Autodesk Inventor part; units mm, degrees
ref_plane "YZ Plane" through (0, 0, 0) normal (1, 0, 0) x (0, 1, 0)
ref_plane "XZ Plane" through (0, 0, 0) normal (0, 1, 0) x (-1, 0, 0)
ref_plane "XY Plane" through (0, 0, 0) normal (0, 0, 1) x (1, 0, 0)
sketch "스케치1" plane through (0, 0, 0) normal (0, 1, 0) x (-1, 0, 0)
  line L0 (0, 0) -> (106, 0)
  line L1 (106, 0) -> (106, -67)
  line L2 (106, -67) -> (0, -67)
  line L3 (0, -67) -> (0, 0)
  circle A0 centre (5, -15) radius 1.1
  circle A1 centre (5, -31) radius 1.1
  circle A2 centre (5, -47) radius 1.1
  circle A3 centre (101, -15) radius 1.1
  circle A4 centre (101, -31) radius 1.1
  circle A5 centre (101, -47) radius 1.1
  dimension "d1" = 2.2
  dimension "d4" = 16
  dimension "d7" = 96
  dimension "d10" = 5
  dimension "d11" = 15
  dimension "d12" = 5
  dimension "d13" = 20
extrude "돌출1" add sketch "스케치1" along normal blind 5
sketch "스케치2" plane through (0, 5, 0) normal (0, 1, 0) x (1, 0, 0)
  circle A0 centre (-5, 15) radius 1.1
  circle A1 centre (-5, 15) radius 2.1
  circle A2 centre (-5, 31) radius 1.1
  circle A3 centre (-5, 31) radius 2.1
  circle A4 centre (-5, 47) radius 1.1
  circle A5 centre (-5, 47) radius 2.1
  circle A6 centre (-101, 47) radius 1.1
  circle A7 centre (-101, 47) radius 2.1
  circle A8 centre (-101, 31) radius 1.1
  circle A9 centre (-101, 31) radius 2.1
  circle A10 centre (-101, 15) radius 1.1
  circle A11 centre (-101, 15) radius 2.1
  point P0 (0, 0)
  dimension "d16" = 4.2
  dimension "d17" = 4.2
  dimension "d18" = 4.2
  dimension "d19" = 4.2
  dimension "d20" = 4.2
  dimension "d21" = 4.2
extrude "돌출2" cut sketch "스케치2" against normal blind 3
sketch "스케치3" plane through (0, 5, 0) normal (0, 1, 0) x (1, 0, 0)
  line L0 (-106, 67) -> (0, 67)
  line L1 (-106, 0) -> (0, 0)
  line L2 (-91, 67) -> (-15, 67)
  line L3 (-15, 67) -> (-15, 0)
  line L4 (-15, 0) -> (-91, 0)
  line L5 (-91, 0) -> (-91, 67)
  line L6 (0, 0) -> (0, 67)
  line L7 (-106, 67) -> (-106, 0)
  line L8 (-91, 0) -> (-15, 0)
  line L9 (-15, 0) -> (-15, 5)
  line L10 (-15, 5) -> (-91, 5)
  line L11 (-91, 5) -> (-91, 0)
  line L12 (-91, 55) -> (-15, 55)
  line L13 (-15, 55) -> (-15, 50)
  line L14 (-15, 50) -> (-91, 50)
  line L15 (-91, 50) -> (-91, 55)
  dimension "d24" = 15
  dimension "d25" = 15
  dimension "d26" = 5
  dimension "d27" = 5
  dimension "d30" = 45
extrude "돌출3" add sketch "스케치3" along normal blind 60 contours L12 L3 L14 L5 | L5 L10 L3 L1
sketch "스케치4" plane through (-106, 0, 0) normal (0, 0, 1) x (1, 0, 0)
  circle A0 centre (53, 60) radius 1.1
  circle A1 centre (77, 60) radius 1.1
  circle A2 centre (29, 60) radius 1.1
  line L0 (91, 5) -> (91, 65)
  line L1 (15, 65) -> (91, 65)
  point P0 (106, 0)
  dimension "d33" = 2.2
  dimension "d34" = 2.2
  dimension "d35" = 2.2
  dimension "d36" = 24
  dimension "d37" = 24
  dimension "d38" = 38
  dimension "d39" = 5
  dimension "d40" = 5
  dimension "d41" = 5
extrude "돌출4" cut sketch "스케치4" against normal blind 55
sketch "스케치5" plane through (-106, 0, 0) normal (0, 0, 1) x (1, 0, 0)
  circle A0 centre (29, 60) radius 1.1
  circle A1 centre (29, 60) radius 2.1
  circle A2 centre (53, 60) radius 1.1
  circle A3 centre (53, 60) radius 2.1
  circle A4 centre (77, 60) radius 1.1
  circle A5 centre (77, 60) radius 2.1
  point P0 (106, 0)
  dimension "d44" = 4.2
  dimension "d45" = 4.2
  dimension "d46" = 4.2
sketch "스케치6" plane through (-15, 5, -55) normal (0, 0, -1) x (-1, 0, 0)
  circle A0 centre (14, 55) radius 1.1
  circle A1 centre (14, 55) radius 2.1
  circle A2 centre (38, 55) radius 1.1
  circle A3 centre (38, 55) radius 2.1
  circle A4 centre (62, 55) radius 1.1
  circle A5 centre (62, 55) radius 2.1
  point P0 (-15, -5)
  dimension "d47" = 4.2
  dimension "d48" = 4.2
  dimension "d49" = 4.2
extrude "돌출5" cut sketch "스케치6" against normal blind 3
extrude "돌출6" cut sketch "스케치5" against normal blind 3
sketch "스케치7" plane through (0, 5, 0) normal (0, 1, 0) x (1, 0, 0)
  line L0 (-91, 67) -> (-15, 67)
  line L1 (-15, 67) -> (-15, 64.3)
  line L2 (-15, 64.3) -> (-91, 64.3)
  line L3 (-91, 64.3) -> (-91, 67)
  line L4 (-91, 55) -> (-91, 50)
  line L5 (-15, 50) -> (-15, 55)
  line L6 (-15, 55) -> (-91, 55)
  line L7 (-126.75, 50) -> (-121.75, 50)
  line L8 (-121.75, 50) -> (-121.75, 67)
  line L9 (-121.75, 67) -> (-126.75, 67)
  line L10 (-126.75, 67) -> (-126.75, 50)
  line L11 (15.75, 50) -> (20.75, 50)
  line L12 (20.75, 50) -> (20.75, 67)
  line L13 (20.75, 67) -> (15.75, 67)
  line L14 (15.75, 67) -> (15.75, 50)
  line L15 (-106, 67) -> (-106, 0)
  line L16 (-126.75, 50) -> (-106, 50)
  line L17 (-106, 50) -> (-106, 67)
  line L18 (-106, 67) -> (-126.75, 67)
  line L19 (-126.75, 67) -> (-126.75, 50)
  line L20 (0, 50) -> (20.75, 50)
  line L21 (20.75, 50) -> (20.75, 67)
  line L22 (20.75, 67) -> (0, 67)
  line L23 (0, 67) -> (0, 50)
  point P0 (0, 0)
  point P1 (0, 67)
  dimension "d54" = 9.3
  dimension "d56" = 5
  dimension "d57" = 5
  dimension "d58" = 137.5
  dimension "d59" = 15.75
extrude "돌출7" add sketch "스케치7" along normal blind 40 contours L10 L9 L8 L7 | L14 L13 L12 L11
extrude "돌출8" add sketch "스케치7" against normal blind 5 contours L10 L9 L8 L7 | L8 L18 L15 L16 | L14 L13 L12 L11 | L20 L23 L22 L14
extrude "돌출9" add sketch "스케치7" along normal blind 40 contours L0 L1 L2 L3
sketch "스케치8" plane through (15.75, 5, -67) normal (-1, 0, 0) x (0, 0, 1)
  line L0 (17, 0) -> (12, 0)
  line L1 (17, 0) -> (12, 0)
  line L2 (12, 0) -> (12, 40)
  line L3 (12, 40) -> (17, 40)
  line L4 (17, 40) -> (17, 0)
  point P0 (67, -5)
  dimension "d66" = 5
  dimension "d67" = 40
extrude "돌출10" add sketch "스케치8" along normal blind 142.5
sketch "스케치9" plane through (0, 5, 0) normal (0, 1, 0) x (1, 0, 0)
  line L0 (0, 50) -> (-106, 50)
  line L1 (-94, 5) -> (-12, 5)
  line L2 (-12, 5) -> (-12, 50)
  line L3 (-12, 50) -> (-94, 50)
  line L4 (-94, 50) -> (-94, 5)
  line L5 (-15, 5) -> (-91, 5)
  line L6 (-106, 50) -> (-106, 0)
  line L7 (0, 0) -> (0, 50)
  dimension "d70" = 12
  dimension "d71" = 12
extrude "돌출11" cut sketch "스케치9" against normal blind 10
equation "\"d25\" = d24"
properties part number "Frame"
Design review of the part built by this model. Coordinates are the model's own, in mm. A direction names the side the tool comes from. Give positions to 0.01 mm unless a question says otherwise; leave off trailing zeros. Order: outer loops, then holes, each group sorted by start corner. A loop starts at its lowest first (then second) coordinate and runs counter-clockwise, first axis right, second up. Notation, with made-up numbers: (-22.5, 24) -> (18.5, 24) arc R23 ccw to (18.5, 49) -> close; hole circle Ø6 at (-26, 35.25). An arc over 180 degrees is marked (long way). Write item = value, one per line. Start each with the question number.
(1) We need section B-B on x = -18.5. Write out the cut boundary in (y, z), plus the area to 3 significant figures.
(2) We need section C-C on z = -7.5. Write out the cut boundary in (x, y), plus the area to 3 significant figures.
(3) We need section A-A on y = 20.5. Write out the cut boundary in (x, z).
(4) For faces 4 (the face through (-5.46, 3.52, -28.95)), 5 (the face through (0, 2, -25)), 6 (the face through (-27.334, 58.722, -53.521)), list the 3-axis set-ups (+Z, -Z, +X, -X, +Y, -Y) from which the entire face can be reached by the end or side of a thin tool; tool diameter is ignored.
(5) Mouldability with a two-part tool opening along Z and no side actions: class faces 1 (the face through (-54, 22, -67)), 2 (the face through (-103.1, 3.52, -31.09)), 3 (the face through (-52.031, 58.137, -1.479)) as +Z half, -Z half, draft (parallel to the pull), parting line (faces both ways), or undercut.
(6) We need section D-D on y = 50. Write out the cut boundary in (x, z).
(7) For pin 1 (4 mm diameter, centred on x = -77, y = 60, fed in from +Z); pin 2 (3.5 mm diameter, centred on x = -29, y = 60, fed in from -Z); pin 3 (1.5 mm diameter, centred on x = -3.5, y = 38, fed in from -Z), all flat-tipped, find the tip position at first contact; note any pin that passes through.
(8) To check wall thickness, follow line 1 along Z through (x, y) = (-75, 32); line 2 along Z through (x, y) = (-101, 1.2); line 3 along X through (y, z) = (60, -51.4). State the ranges of each line that lie inside material, in increasing order.
Numbers:
q1.outline = (0, -67) -> (45, -67) -> (45, -64.3) -> (5, -64.3) -> (5, -55) -> (65, -55) -> (65, -50) -> (0, -50) -> close; (0, -5) -> (65, -5) -> (65, 0) -> (0, 0) -> close
q1.area = 818 mm^2
q2.outline = (-106, 0) -> (-94, 0) -> (-94, 5) -> (-106, 5) -> close; (-12, 0) -> (0, 0) -> (0, 5) -> (-12, 5) -> close
q2.area = 120 mm^2
q3.outline = (-126.75, -67) -> (-121.75, -67) -> (-121.75, -55) -> (15.75, -55) -> (15.75, -67) -> (20.75, -67) -> (20.75, -50) -> (-126.75, -50) -> close; (-91, -67) -> (-15, -67) -> (-15, -64.3) -> (-91, -64.3) -> close; (-91, -5) -> (-15, -5) -> (-15, 0) -> (-91, 0) -> close
q4.face_4 = +Y
q4.face_5 = +Z, +X, +Y, -Y
q4.face_6 = -Z
q5.face_1 = -Z half
q5.face_2 = undercut
q5.face_3 = draft
q6.outline = (-91, -55) -> (-15, -55) -> (-15, -50) -> (-91, -50) -> close; (-91, -5) -> (-15, -5) -> (-15, 0) -> (-91, 0) -> close
q7.pin_1 = -3
q7.pin_2 = -52
q7.pin_3 = -55
q8.line_1 = -67 to -64.3, -55 to -50, -5 to 0
q8.line_2 = -67 to -48.1, -45.9 to -32.1, -29.9 to -16.1, -13.9 to 0
q8.line_3 = -91 to -78.1, -75.9 to -54.1, -51.9 to -30.1, -27.9 to -15
